Input: part model. Units: mm. Frame: model coordinates. A direction names the side the tool comes from. Round coordinates to 2 decimals unless told otherwise and drop trailing zeros. Loops run counter-clockwise (first coordinate to the right, second up) from the corner with the lowest first, then second, coordinate; pieces in that order, holes last.
1) Section B-B, the plane y = -7.65. Return loops of the section in (x, z).
2) Draft query along Y for faces 5 (the face through (4.54, 5.77, 1.01)), 6 (the face through (5.008, -8.626, 0.542)), 7 (the face through (17.273, -24.086, 1.014)). Return one class per face: pulls with the +Y half, pulls with the -Y half, needs draft (parallel to the pull), parting line crosses it, or undercut.
3) Ray query, line 1 along Y through (x, z) = (23, 1.4); line 2 along Y through (x, z) = (-22.65, 1.1); line 3 along Y through (x, z) = (-5, 1.3). Return the intervals inside material, ascending.
4) Section C-C, the plane x = 4.5. Return loops of the section in (y, z), and give its area (3 significant figures).
5) Section D-D, the plane y = 13. Return loops of the section in (x, z).
6) Access query for faces 1 (the face through (22.713, 19.265, 1.014)), 2 (the face through (-10.91, -17.94, 0.99)), 3 (the face through (-15.08, -13.62, 0.99)), 4 (the face through (11.51, 14.53, 0.99)). Directions: +Z, -Z, +X, -X, +Y, -Y. A direction counts if a zero-diameter tool reaches every point of the face in a straight line with its end or side. Return the directions, or none.
7) First-contact query: pin 1 (3 mm diameter, centred on x = 4.5, y = -7.65, fed in from +Z); pin 2 (0.6 mm diameter, centred on y = -2.5, z = 1, fed in from +X); pin 3 (1 mm diameter, centred on x = -1, z = 1, fed in from +Y). Flat tips, straight axial feed; report the tip coordinate or a pass-through.
8) Section A-A, the plane x = -10.5. Return loops of the section in (y, z), and give its area (3 significant figures).
from build123d import *

# Parameters (mm, degrees)
F1_R     = 2.85
F1_R_2   = 1.1
F2_DEPTH = 2
F3_R     = 4
F4_SIZE  = 0.9


with BuildPart() as f2:
    # F1 (on Top) → F2 (new body)
    with BuildSketch(Plane.XY):
        with BuildLine():
            Line((-8.5, -7.576114), (-21.734057, -19.734611))
            ThreePointArc((-21.734057, -19.734611), (-26.331988, -28.032745), (-17.674763, -24.152997))
            Line((-17.674763, -24.152997), (-4.065732, -11.65))
            Line((-4.065732, -11.65), (4.065732, -11.65))
            Line((4.065732, -11.65), (17.674763, -24.152997))
            ThreePointArc((17.674763, -24.152997), (26.331988, -28.032745), (21.734057, -19.734611))
            Line((21.734057, -19.734611), (8.5, -7.576114))
            Line((8.5, -7.576114), (8.5, 0.276202))
            Line((8.5, 0.276202), (22.704322, 19.650295))
            ThreePointArc((22.704322, 19.650295), (25.606365, 28.682357), (17.865493, 23.197934))
            Line((17.865493, 23.197934), (4.780091, 5.35))
            Line((4.780091, 5.35), (-4.780091, 5.35))
            Line((-4.780091, 5.35), (-17.865493, 23.197934))
            ThreePointArc((-17.865493, 23.197934), (-25.606365, 28.682357), (-22.704322, 19.650295))
            Line((-22.704322, 19.650295), (-8.5, 0.276202))
            Line((-8.5, 0.276202), (-8.5, -7.576114))
        make_face()
        with Locations((-22.65, -24.65)):
            Circle(F1_R, mode=Mode.SUBTRACT)
        with Locations((-4.5, -7.65)):
            Circle(F1_R_2, mode=Mode.SUBTRACT)
        with Locations((22.65, -24.65)):
            Circle(F1_R, mode=Mode.SUBTRACT)
        with Locations((4.5, -7.65)):
            Circle(F1_R_2, mode=Mode.SUBTRACT)
        with Locations((-4.5, 1.35)):
            Circle(F1_R_2, mode=Mode.SUBTRACT)
        with Locations((-22.65, 24.65)):
            Circle(F1_R, mode=Mode.SUBTRACT)
        with Locations((4.5, 1.35)):
            Circle(F1_R_2, mode=Mode.SUBTRACT)
        with Locations((22.65, 24.65)):
            Circle(F1_R, mode=Mode.SUBTRACT)
    extrude(amount=F2_DEPTH)

    # F3
    f3_edges = [f2.edges().sort_by_distance(p)[0] for p in [
        (-22.704322, 19.650295, 1),
        (-8.5, 0.276202, 1),
        (-8.5, -7.576114, 1),
        (-21.734057, -19.734611, 1),
        (-17.674763, -24.152997, 1),
        (-4.065732, -11.65, 1),
        (4.065732, -11.65, 1),
        (17.674763, -24.152997, 1),
        (21.734057, -19.734611, 1),
        (8.5, -7.576114, 1),
        (8.5, 0.276202, 1),
        (22.704322, 19.650295, 1),
        (17.865493, 23.197934, 1),
        (4.780091, 5.35, 1),
        (-4.780091, 5.35, 1),
        (-17.865493, 23.197934, 1),
    ]]
    fillet(f3_edges, radius=F3_R)

    # F4
    f4_edges = [f2.edges().sort_by_distance(p)[0] for p in [
        (-5.6, 1.35, 2),
        (3.4, 1.35, 2),
        (3.4, -7.65, 2),
        (-5.6, -7.65, 2),
    ]]
    chamfer(f4_edges, length=F4_SIZE)


solid = f2.part
Final values:
1. outline: (-8.94, 0) - (-5.6, 0) - (-5.6, 1.1) - (-6.5, 2) - (-8.94, 2) - close; (-3.4, 0) - (3.4, 0) - (3.4, 1.1) - (2.5, 2) - (-2.5, 2) - (-3.4, 1.1) - close; (5.6, 0) - (8.94, 0) - (8.94, 2) - (6.5, 2) - (5.6, 1.1) - close
2. face 5: pulls with the +Y half
2. face 6: undercut
2. face 7: pulls with the -Y half
3. line 1: y = -29.64 to -27.48, -21.82 to -19.66, 19.44 to 21.82, 27.48 to 29.64
3. line 2: y = -29.65 to -27.5, -21.8 to -19.63, 19.22 to 21.8, 27.5 to 29.65
3. line 3: y = -12.52 to -8.85, -6.45 to 0.15, 2.55 to 6.04
4. outline: (-12.18, 0) - (-8.75, 0) - (-8.75, 1.1) - (-9.65, 2) - (-12.18, 2) - close; (-6.55, 0) - (0.25, 0) - (0.25, 1.1) - (-0.65, 2) - (-5.65, 2) - (-6.55, 1.1) - close; (2.45, 0) - (5.75, 0) - (5.75, 2) - (3.35, 2) - (2.45, 1.1) - close
4. area: 25.4 mm2
5. outline: (-17.83, 0) - (-10.39, 0) - (-10.39, 2) - (-17.83, 2) - close; (10.39, 0) - (17.83, 0) - (17.83, 2) - (10.39, 2) - close
6. face 1: +Z, -Z, +X
6. face 2: +Z, -Z, -Y
6. face 3: +Z, -Z, -X
6. face 4: +Z, -Z, +Y
7. pin 1: stops at z = 1.5
7. pin 2: stops at x = 8.5
7. pin 3: stops at y = 5.35
8. outline: (-17.56, 0) - (-9.41, 0) - (-9.41, 2) - (-17.56, 2) - close; (3, 0) - (13.15, 0) - (13.15, 2) - (3, 2) - close
8. area: 36.6 mm2
